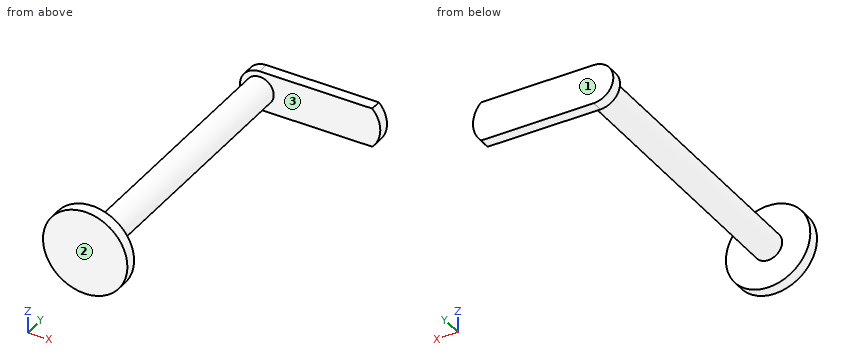
from build123d import *

# Parameters (mm, degrees)
SKETCH1_R           = 6.35
BOSS_EXTRUDE2_DEPTH = 127
SKETCH2_R           = 8.89
BOSS_EXTRUDE3_DEPTH = 5.08
BOSS_EXTRUDE5_DEPTH = 5.08
SKETCH4_R           = 19.05
BOSS_EXTRUDE6_DEPTH = 5.08


with BuildPart() as part:
    # Sketch1 → Boss-Extrude2 (new body)
    with BuildSketch(Plane(origin=(0, 0, 0), x_dir=(1, 0, 0), z_dir=(0, 1, 0))):
        with Locations(Location((0, 0, 0), (0, 0, 270))):
            Circle(SKETCH1_R)
    extrude(amount=BOSS_EXTRUDE2_DEPTH)

    # Sketch2 → Boss-Extrude3 (add)
    with BuildSketch(Plane(origin=(0, 127, 0), x_dir=(1, 0, 0), z_dir=(0, 1, 0))):
        with Locations(Location((0, 0, 0), (0, 0, 270))):
            Circle(SKETCH2_R)
    extrude(amount=BOSS_EXTRUDE3_DEPTH)

    # Sketch3 → Boss-Extrude5 (add)
    with BuildSketch(Plane(origin=(0, 132.08, 0), x_dir=(1, 0, 0), z_dir=(0, 1, 0))):
        with BuildLine():
            Line((0, 8.89), (50.8, 8.89))
            ThreePointArc((50.8, 8.89), (54.430385896, 0), (50.8, -8.89))
            Line((50.8, -8.89), (0, -8.89))
            Line((0, -8.89), (0, 8.89))
        make_face()
    extrude(amount=-BOSS_EXTRUDE5_DEPTH)

    # Sketch4 → Boss-Extrude6 (add)
    with BuildSketch(Plane.XZ):
        with Locations(Location((0, 0, 0), (0, 0, 270))):
            Circle(SKETCH4_R)
    extrude(amount=BOSS_EXTRUDE6_DEPTH)


solid = part.part
Design review of the part built by this model. Coordinates are the model's own, in mm. Face numbers are marked on the shaded views. Give positions to 0.01 mm unless a question says otherwise; leave off trailing zeros. Order: outer loops, then holes, each group sorted by start corner. A loop starts at its lowest first (then second) coordinate and runs counter-clockwise, first axis right, second up. Notation, with made-up numbers: (-3.5, -27) - (5.5, -27) arc R17 ccw to (5.5, -20) - close; hole circle Ø7 at (58.5, 82.25). An arc over 180 degrees is marked (long way). Write item = value, one per line. Start each with the question number.
Q1. Mouldability with a two-part tool opening along Y and no side actions: class the marked faces 1, 2 and 3 as released by +Y, released by -Y, zero draft, split by the parting line, or undercut.
Q2. We need section C-C on x = 29.5. State the section outline as (y, z) points, plus the area to 3 significant figures.
Q3. We need section D-D on y = 72. State the section outline as (x, z) points, plus the area to 3 significant figures.
Q4. We need section A-A on z = 0. State the section outline as (x, y) points, plus the area to 3 significant figures.
Q5. We need section B-B on x = 10. State the section outline as (y, z) points, plus the area to 3 significant figures.
Q6. Clearance check with flat-ended pins moving along their axes: pin 1 Ø2.5 at (x, y) = (35.5, 130.5) entering from +Z; pin 2 Ø12 at (x, z) = (37.5, 10) entering from +Y; pin 3 Ø19.5 at (x, z) = (37.5, 1) entering from -Y; pin 4 Ø8 at (x, y) = (3, 76) entering from -Z. State where each tip first meets the part, or that it passes through.
Q7. To check wall thickness, follow L1, parallel to Y at x = -13.5, z = 1.5; L2, parallel to Y at x = 38.5, z = 1; L3, parallel to X at y = 46.5, z = -5. State the ranges of each line that lie inside material, in increasing order. Write a range as from..to.
Working result:
q1.face_1 = released by +Y
q1.face_2 = released by -Y
q1.face_3 = undercut
q2.outline = (127, -8.89) - (132.08, -8.89) - (132.08, 8.89) - (127, 8.89) - close
q2.area = 90.3 mm²
q3.outline = circle Ø12.7 at (0, 0)
q3.area = 127 mm²
q4.outline = (-19.05, -5.08) - (19.05, -5.08) - (19.05, 0) - (6.35, 0) - (6.35, 127) - (54.43, 127) - (54.43, 132.08) - (-8.89, 132.08) - (-8.89, 127) - (-6.35, 127) - (-6.35, 0) - (-19.05, 0) - close
q4.area = 2,130 mm²
q5.outline = (-5.08, -16.21) - (0, -16.21) - (0, 16.21) - (-5.08, 16.21) - close; (127, -8.89) - (132.08, -8.89) - (132.08, 8.89) - (127, 8.89) - close
q5.area = 255 mm²
q6.pin_1 = 8.89
q6.pin_2 = 132.08
q6.pin_3 = 127
q6.pin_4 = -6.35
q7.L1 = -5.08..0
q7.L2 = 127..132.08
q7.L3 = -3.91..3.91
